Design review of the part built by this model. Coordinates are the model's own, in mm. A direction names the side the tool comes from. Coordinates: 2 decimals unless noted, no trailing zeros. Loops run counter-clockwise (first coordinate to the right, second up) from the corner with the lowest first, then second, coordinate; pieces in that order, holes last.
Q1. Add section D-D on z = -8. Give the boundary of the cut face in (x, y).
Q2. For P1, Ø10, axis at x = 18, z = 7, coming from the +Y side; P2, Ø4, axis at x = 18, z = -6, coming from the -Y side; P3, Ø6, axis at x = 24, y = -6.5, coming from the +Z side; P4, Ø3, axis at y = 6, z = -4, coming from the +X side, all flat-tipped, find the tip position at first contact; note any pin that passes through.
Q3. Add section A-A on x = 3.5. Give the boundary of the cut face in (y, z), and give its area (3 significant figures).
Q4. Add section C-C on z = -0.75. Give the boundary of the cut face in (x, y), and give its area (3 significant figures).
Q5. Wall thickness on probe 1 along X at (y, z) = (-2.5, -0.75); probe 2 along Y at (x, z) = (19, 8.5); probe 3 along X at (y, z) = (-1.5, -6.25): over which ranges is each line inside the solid? List them lowest first.
Q6. Machinability: for faces 4 (the face through (26, 0, 1.25)), 5 (the face through (24.95, 4.77, 1.5)), 6 (the face through (10.6, 0, 9.4)), which of the approach directions +Z, -Z, +X, -X, +Y, -Y give a long, thin tool a straight path to every point of the face, cutting with its end or side? Answer none if there is none.
Q7. Draft analysis for pull direction Z (two halves, no side actions). For faces 1 (the face through (10.6, 3.75, -3.86)), 2 (the face through (23.5, 0, 0)), 3 (the face through (29, 0, -2)), state which applies: released by +Z, released by -Z, zero draft, split by the parting line, or undercut.
Q8. Add section B-B on y = 0. Give the boundary of the cut face in (x, z), and give its area (3 significant figures).
```python
from build123d import *

# Parameters (mm, degrees)
F1_DEPTH = 21.5
F2_R     = 5
F3_DEPTH = 7.5
F4_SIZE  = 0.5
F6_DEPTH = 5.5


with BuildPart() as f1:
    # F0 (on Right) → F1 (new body)
    with BuildSketch(Plane.YZ):
        with BuildLine():
            ThreePointArc((-1.1652526978, 8.4866812693), (-0.1443896855, 7.0087184973), (1.2, 8.2))
            ThreePointArc((1.2, 8.2), (1.1912815027, 8.3443896855), (1.1652526978, 8.4866812693))
            ThreePointArc((1.1652526978, 8.4866812693), (0, 9.4), (-1.1652526978, 8.4866812693))
        make_face()
        with BuildLine():
            ThreePointArc((1.1652526978, 8.4866812693), (1.1912815027, 8.3443896855), (1.2, 8.2))
            ThreePointArc((1.2, 8.2), (-0.1443896855, 7.0087184973), (-1.1652526978, 8.4866812693))
            ThreePointArc((-1.1652526978, 8.4866812693), (-3.8046240347, 3.8046240347), (-8.4866812693, 1.1652526978))
            ThreePointArc((-8.4866812693, 1.1652526978), (-7.4597356969, 0.9444621547), (-7, 0))
            ThreePointArc((-7, 0), (-7.4597356969, -0.9444621547), (-8.4866812693, -1.1652526978))
            ThreePointArc((-8.4866812693, -1.1652526978), (-3.8046240347, -3.8046240347), (-1.1652526978, -8.4866812693))
            ThreePointArc((-1.1652526978, -8.4866812693), (-0.1443896855, -7.0087184973), (1.2, -8.2))
            ThreePointArc((1.2, -8.2), (1.1912815027, -8.3443896855), (1.1652526978, -8.4866812693))
            ThreePointArc((1.1652526978, -8.4866812693), (3.8046240347, -3.8046240347), (8.4866812693, -1.1652526978))
            ThreePointArc((8.4866812693, -1.1652526978), (7, 0), (8.4866812693, 1.1652526978))
            ThreePointArc((8.4866812693, 1.1652526978), (3.8046240347, 3.8046240347), (1.1652526978, 8.4866812693))
        make_face()
        with BuildLine():
            ThreePointArc((9.4, 0), (9.1444621547, 0.7402643031), (8.4866812693, 1.1652526978))
            ThreePointArc((8.4866812693, 1.1652526978), (7, 0), (8.4866812693, -1.1652526978))
            ThreePointArc((8.4866812693, -1.1652526978), (9.1444621547, -0.7402643031), (9.4, 0))
        make_face()
        with BuildLine():
            ThreePointArc((-7, 0), (-7.4597356969, 0.9444621547), (-8.4866812693, 1.1652526978))
            ThreePointArc((-8.4866812693, 1.1652526978), (-9.4, 0), (-8.4866812693, -1.1652526978))
            ThreePointArc((-8.4866812693, -1.1652526978), (-7.4597356969, -0.9444621547), (-7, 0))
        make_face()
        with BuildLine():
            ThreePointArc((-1.1652526978, -8.4866812693), (0, -9.4), (1.1652526978, -8.4866812693))
            ThreePointArc((1.1652526978, -8.4866812693), (1.1912815027, -8.3443896855), (1.2, -8.2))
            ThreePointArc((1.2, -8.2), (-0.1443896855, -7.0087184973), (-1.1652526978, -8.4866812693))
        make_face()
    extrude(amount=F1_DEPTH)

    # F2 (on face) → F3 (join)
    with BuildSketch(Plane.YZ.offset(21.5)):
        Circle(F2_R)
    extrude(amount=F3_DEPTH)

    # F4
    f4_edges = [f1.edges().sort_by_distance(p)[0] for p in [
        (29, -5, 0),
    ]]
    chamfer(f4_edges, length=F4_SIZE)

    # F5 (on face) → F6 (cut)
    with BuildSketch(Plane.YZ.offset(29)):
        with BuildLine():
            ThreePointArc((4.5, 0), (4.4555060613, 0.6312414261), (4.3229041164, 1.25))
            Line((4.3229041164, 1.25), (-4.3229041164, 1.25))
            ThreePointArc((-4.3229041164, 1.25), (-4.5, 0), (-4.3229041164, -1.25))
            Line((-4.3229041164, -1.25), (4.3229041164, -1.25))
            ThreePointArc((4.3229041164, -1.25), (4.4555060613, -0.6312414261), (4.5, 0))
        make_face()
        with BuildLine():
            Line((-4.3229041164, 1.25), (-4.8412291828, 1.25))
            ThreePointArc((-4.8412291828, 1.25), (-5, 0), (-4.8412291828, -1.25))
            Line((-4.8412291828, -1.25), (-4.3229041164, -1.25))
            ThreePointArc((-4.3229041164, -1.25), (-4.5, 0), (-4.3229041164, 1.25))
        make_face()
        with BuildLine():
            ThreePointArc((4.8412291828, -1.25), (4.9601484813, -0.6300214624), (5, 0))
            ThreePointArc((5, 0), (4.9601484813, 0.6300214624), (4.8412291828, 1.25))
            Line((4.8412291828, 1.25), (4.3229041164, 1.25))
            ThreePointArc((4.3229041164, 1.25), (4.4555060613, 0.6312414261), (4.5, 0))
            ThreePointArc((4.5, 0), (4.4555060613, -0.6312414261), (4.3229041164, -1.25))
            Line((4.3229041164, -1.25), (4.8412291828, -1.25))
        make_face()
    extrude(amount=-F6_DEPTH, mode=Mode.SUBTRACT)


solid = f1.part
```
Entries:
1. outline: (0, -1.3) - (21.5, -1.3) - (21.5, 1.3) - (0, 1.3) - close
2. P1: stops at y = 6.27
2. P2: stops at y = -3.61
2. P3: stops at z = 3.57
2. P4: passes through
3. outline: (-8.49, -1.17) arc R10 cw to (-1.17, -8.49) arc R1.2 ccw to (1.17, -8.49) arc R10 cw to (8.49, -1.17) arc R1.2 ccw to (8.49, 1.17) arc R10 cw to (1.17, 8.49) arc R1.2 ccw to (-1.17, 8.49) arc R10 cw to (-8.49, 1.17) arc R1.2 ccw to start
3. area: 147 mm2
4. outline: (0, -9.14) - (21.5, -9.14) - (21.5, -4.94) - (23.5, -4.94) - (23.5, 4.94) - (21.5, 4.94) - (21.5, 9.14) - (0, 9.14) - close
4. area: 413 mm2
5. probe 1: x = 0 to 23.5
5. probe 2: y = -1.16 to 1.16
5. probe 3: x = 0 to 21.5
6. face 4: +X, +Y, -Y
6. face 5: +X
6. face 6: +Z, +X, -X
7. face 1: released by -Z
7. face 2: undercut
7. face 3: zero draft
8. outline: (0, -9.4) - (21.5, -9.4) - (21.5, -5) - (28.5, -5) - (29, -4.5) - (29, -1.25) - (23.5, -1.25) - (23.5, 1.25) - (29, 1.25) - (29, 4.5) - (28.5, 5) - (21.5, 5) - (21.5, 9.4) - (0, 9.4) - close
8. area: 465 mm2
